Work out the finished part from the listing and answer in its coordinate system (mm). Face numbers are marked on the shaded views. Coordinates: 2 decimals unless noted, no trailing zeros. Order: outer loops, then holes, each group sorted by start corner. A loop starts at its lowest first (then second) coordinate and runs counter-clockwise, first axis right, second up. Notation, with made-up numbers: (-8.5, 51) -> (22.5, 51) arc R19 cw to (22.5, 61) -> close; hole circle Ø8 at (52, -36). An arc over 180 degrees is marked (long way). Answer as CSV lines item,"result". Start each with the question number.
Item 1: Section A-A (x = 0) is taken. Write down the section's boundary in (y, z), then the cut area to 3 significant figures.
Item 2: Each of these flat-tipped pins is pushed along its axis until it touches: pin 1 Ø0.8 at (y, z) = (-13, 4) entering from +X; pin 2 Ø19.5 at (x, y) = (9.5, 6.5) entering from +Z; pin 3 Ø5 at (x, y) = (12, -12.5) entering from +Z; pin 4 Ø0.7 at (x, y) = (-5.5, -13.5) entering from +Z. Where does it stop, or does it pass through?
Item 3: For a pull along Y with two mould halves and no side action, classify the marked faces 1 and 2 as pulls with the +Y half, pulls with the -Y half, needs draft (parallel to the pull), parting line crosses it, or undercut.
Item 4: Straight lines are drawn through the part: L1, parallel to Z at x = -1, y = -16; L2, parallel to Y at x = 0, z = 1.6; L3, parallel to Z at x = 6, y = 0. For each, find the intervals that lie inside material, in ascending order.
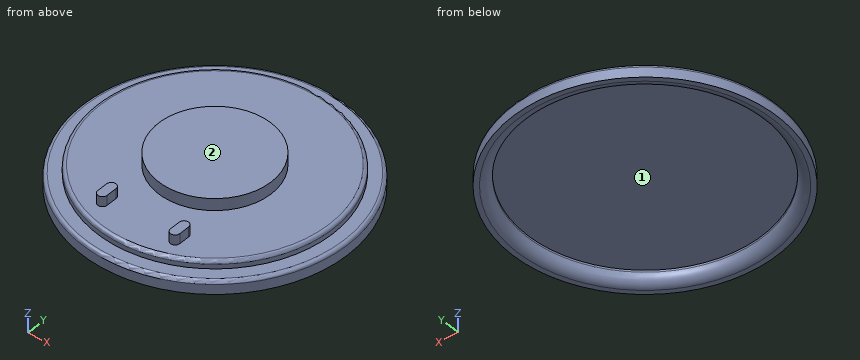
```python
from build123d import *

# Parameters (mm, degrees)
SKETCH_1_R          = 20
EXTRUDE_1_DEPTH     = 5
SKETCH_2_OUTSIDE_W  = 53.358
SKETCH_2_OUTSIDE_H  = 53.358
SKETCH_2_OUTSIDE_R  = 17.75
CUT_EXTRUDE_1_DEPTH = 3
SKETCH_3_OUTSIDE_W  = 53.358
SKETCH_3_OUTSIDE_H  = 53.358
SKETCH_3_OUTSIDE_R  = 8.5
CUT_EXTRUDE_2_DEPTH = 1.8
CUT_EXTRUDE_START   = -1.8
SKETCH_4_R          = 17.75
CUT_EXTRUDE_3_DEPTH = 1.8
FILLET_1_R          = 1.5
FILLET_2_R          = 0.5
FILLET_3_R          = 0.5
EXTRUDE_999_DEPTH   = 1.5


with BuildPart() as part:
    # 草图1 → 拉伸1 (new body)
    with BuildSketch(Plane.XY):
        Circle(SKETCH_1_R)
    extrude(amount=EXTRUDE_1_DEPTH)

    # 草图2 outside → 切除-拉伸1 (cut)
    with BuildSketch(Plane.XY.offset(5)):
        Rectangle(SKETCH_2_OUTSIDE_W, SKETCH_2_OUTSIDE_H)
        Circle(SKETCH_2_OUTSIDE_R, mode=Mode.SUBTRACT)
    extrude(amount=-CUT_EXTRUDE_1_DEPTH, mode=Mode.SUBTRACT)

    # 草图3 outside → 切除-拉伸2 (cut)
    with BuildSketch(Plane.XY.offset(5)):
        Rectangle(SKETCH_3_OUTSIDE_W, SKETCH_3_OUTSIDE_H)
        Circle(SKETCH_3_OUTSIDE_R, mode=Mode.SUBTRACT)
    extrude(amount=-CUT_EXTRUDE_2_DEPTH, mode=Mode.SUBTRACT)

    # 草图4 → 切除-拉伸3 (cut)
    with BuildSketch(Plane(origin=(0, 0, 0), x_dir=(-1, 0, 0), z_dir=(0, 0, -1)).offset(CUT_EXTRUDE_START)):
        with Locations(Location((0, 0, 0), (0, 0, 180))):
            Circle(SKETCH_4_R)
    extrude(amount=CUT_EXTRUDE_3_DEPTH, mode=Mode.SUBTRACT)

    # 圆角1
    fillet_1_edges = [part.edges().sort_by_distance(p)[0] for p in [
        (-17.75, 0, 0),
    ]]
    fillet(fillet_1_edges, radius=FILLET_1_R)

    # 圆角2
    fillet_2_edges = [part.edges().sort_by_distance(p)[0] for p in [
        (-20, 0, 2),
    ]]
    fillet(fillet_2_edges, radius=FILLET_2_R)

    # 圆角3
    fillet_3_edges = [part.edges().sort_by_distance(p)[0] for p in [
        (-17.75, 0, 3.2),
    ]]
    fillet(fillet_3_edges, radius=FILLET_3_R)

    # 草图5 → Extrude 999 (add)
    with BuildSketch(Plane.XY.offset(3.2)):
        with BuildLine():
            Line((-4.8, -12.2), (-4.8, -13.8))
            ThreePointArc((-4.8, -13.8), (-5.5, -14.5), (-6.2, -13.8))
            Line((-6.2, -13.8), (-6.2, -12.2))
            ThreePointArc((-6.2, -12.2), (-5.5, -11.5), (-4.8, -12.2))
        make_face()
        with BuildLine():
            Line((4.8, -12.2), (4.8, -13.8))
            ThreePointArc((4.8, -13.8), (5.5, -14.5), (6.2, -13.8))
            Line((6.2, -13.8), (6.2, -12.2))
            ThreePointArc((6.2, -12.2), (5.5, -11.5), (4.8, -12.2))
        make_face()
    extrude(amount=EXTRUDE_999_DEPTH)


solid = part.part
```
Checked values:
1,outline,"(-20, 0) -> (-19.25, 0) arc R1.5 ccw to (-17.75, 1.5) -> (-17.75, 1.8) -> (17.75, 1.8) -> (17.75, 1.5) arc R1.5 ccw to (19.25, 0) -> (20, 0) -> (20, 1.5) arc R0.5 ccw to (19.5, 2) -> (17.75, 2) -> (17.75, 2.7) arc R0.5 ccw to (17.25, 3.2) -> (8.5, 3.2) -> (8.5, 5) -> (-8.5, 5) -> (-8.5, 3.2) -> (-17.25, 3.2) arc R0.5 ccw to (-17.75, 2.7) -> (-17.75, 2) -> (-19.5, 2) arc R0.5 ccw to (-20, 1.5) -> close"
1,area,"88.1 mm^2"
2,pin 1,"stops at x = 6.2"
2,pin 2,"stops at z = 5"
2,pin 3,"stops at z = 3.2"
2,pin 4,"stops at z = 4.7"
3,face 1,"undercut"
3,face 2,"needs draft"
4,L1,"z = 1.8 to 3.2"
4,L2,"y = -19.99 to -17.75, 17.75 to 19.99"
4,L3,"z = 1.8 to 5"
